from build123d import *

# Parameters (mm, degrees)
BOSS_EXTRUDE1_DEPTH = 11.90625
SKETCH2_R           = 22.225
CUT_EXTRUDE1_DEPTH  = 12.90625


with BuildPart() as part:
    # Sketch1 → Boss-Extrude1 (new body)
    with BuildSketch(Plane.XY):
        Polygon((-337.114930678, -583.900187925), (-216.238948081, -374.536844651), (216.238948081, -374.536844651), (337.114930678, -583.900187925), align=None)
    extrude(amount=-BOSS_EXTRUDE1_DEPTH)

    # Sketch2 → Cut-Extrude1 (cut, through all)
    with BuildSketch(Plane.XY):
        with Locations((-164.309496882, -525.607187925)):
            Circle(SKETCH2_R)
        with Locations((164.309496882, -525.607187925)):
            Circle(SKETCH2_R)
    extrude(amount=-CUT_EXTRUDE1_DEPTH, mode=Mode.SUBTRACT)


solid = part.part
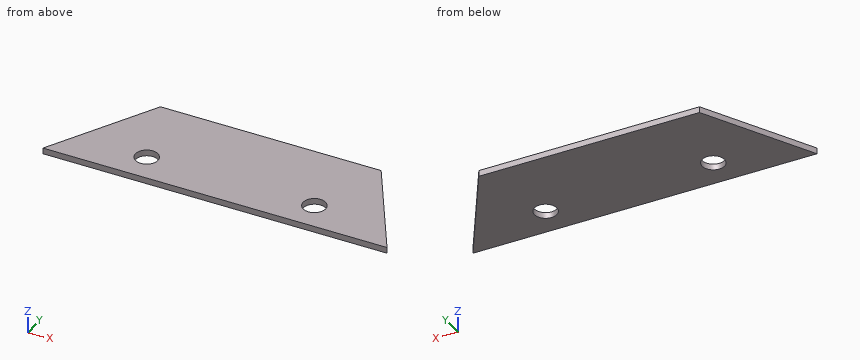
For this review, take the finished solid that the model builds, in its own axes (mm). Round coordinates to 2 decimals unless told otherwise and drop trailing zeros. Loops run counter-clockwise (first coordinate to the right, second up) from the corner with the lowest first, then second, coordinate; pieces in that order, holes last. Notation, with made-up numbers: (85.25, -12) - (139.25, -12) arc R38 ccw to (139.25, 26) - close; hole circle Ø3 at (65, 64.5). An arc over 180 degrees is marked (long way). One line per item, written item: value. Start each with the question number.
Item 1: Clearance check with flat-ended pins moving along their axes: pin 1 Ø1 at (y, z) = (-407.5, -2.5) entering from +X; pin 2 Ø4 at (y, z) = (-474, -10) entering from -X. State where each tip first meets the part, or that it passes through.
Item 2: Take a section at A-A (y = -537.5). Give the boundary of the cut face in (x, z), plus the area to 3 significant figures.
Item 3: Take a section at B-B (z = -2.25). State how many separate pieces and enclosed holes the cut face has, plus the area to 3 significant figures.
Item 4: Take a section at D-D (y = -569.5). Give the boundary of the cut face in (x, z), plus the area to 3 significant figures.
Item 5: Take a section at C-C (x = -252). Give the boundary of the cut face in (y, z).
Item 6: For L1, parallel to X at y = -534, z = -9; L2, parallel to X at y = -541, z = -9.5; L3, parallel to X at y = -394, z = -6.5, list the stretches that pass through material, from the lowest coordinate up.
Answer below:
1. pin 1: stops at x = 235.56
1. pin 2: stops at x = -274.82
2. outline: (-310.33, -11.91) - (-183.08, -11.91) - (-183.08, 0) - (-310.33, 0) - close; (-145.53, -11.91) - (145.53, -11.91) - (145.53, 0) - (-145.53, 0) - close; (183.08, -11.91) - (310.33, -11.91) - (310.33, 0) - (183.08, 0) - close
2. area: 6,500 mm2
3. separate pieces: 1
3. enclosed holes: 2
3. area: 113,000 mm2
4. outline: (-328.8, -11.91) - (328.8, -11.91) - (328.8, 0) - (-328.8, 0) - close
4. area: 7,830 mm2
5. outline: (-583.9, -11.91) - (-436.48, -11.91) - (-436.48, 0) - (-583.9, 0) - close
6. L1: x = -308.31 to -184.89, -143.73 to 143.73, 184.89 to 308.31
6. L2: x = -312.35 to -180.34, -148.28 to 148.28, 180.34 to 312.35
6. L3: x = -227.48 to 227.48
